Read the model definition and answer for the solid it produces. Units are mm, in the model's axes. A direction names the side the tool comes from. Round coordinates to 2 decimals unless told otherwise and drop trailing zeros. Loops run counter-clockwise (first coordinate to the right, second up) from the corner with the lowest first, then second, coordinate; pieces in that order, holes last. Notation, with made-up numbers: (85.25, 19) - (116.25, 19) arc R13 ccw to (116.25, 38) - close; hole circle Ø5 at (80, 77). An arc over 180 degrees is marked (long way). Answer as CSV lines item,"result".
```python
from build123d import *

# Parameters (mm, degrees)
F1_DEPTH = 57
F3_DEPTH = 20
F4_W     = 2.7
F4_H     = 7
F4_W_2   = 27.2
F5_DEPTH = 4.1
F6_DEPTH = 1.9


with BuildPart() as f1:
    # F0 (on Front) → F1 (new body)
    with BuildSketch(Plane.XZ):
        with BuildLine():
            Line((20.8, 15.8), (-20.8, 15.8))
            ThreePointArc((-20.8, 15.8), (-27.871068, 12.871068), (-30.8, 5.8))
            Line((-30.8, 5.8), (-30.8, 0))
            Line((-30.8, 0), (30.8, 0))
            Line((30.8, 0), (30.8, 5.8))
            ThreePointArc((30.8, 5.8), (27.871068, 12.871068), (20.8, 15.8))
        make_face()
    extrude(amount=F1_DEPTH)

    # F2 (on Right) → F3 (join, symmetric)
    with BuildSketch(Plane.YZ):
        with BuildLine():
            Line((0, 15), (0, 0))
            Line((0, 0), (0.6, 0))
            ThreePointArc((0.6, 0), (2.014214, 0.585786), (2.6, 2))
            Line((2.6, 2), (2.6, 13))
            ThreePointArc((2.6, 13), (2.014214, 14.414214), (0.6, 15))
            Line((0.6, 15), (0, 15))
        make_face()
    extrude(amount=F3_DEPTH, both=True)

    # F4 (on face) → F5 (cut)
    with BuildSketch(Plane.XZ.offset(57)):
        with Locations((-15.35, 7.7)):
            Rectangle(F4_W, F4_H)
        with Locations((-0.4, 7.7)):
            Rectangle(F4_W_2, F4_H)
        with Locations((14.55, 7.7)):
            Rectangle(F4_W, F4_H)
    extrude(amount=-F5_DEPTH, mode=Mode.SUBTRACT)

    # F4 (on face) → F6 (join)
    with BuildSketch(Plane.XZ.offset(57)):
        with Locations((-0.4, 7.7)):
            Rectangle(F4_W_2, F4_H)
    extrude(amount=-F6_DEPTH)


solid = f1.part
```
1) A cutting plane is placed at B-B, the plane z = 9.75. Determine the outline of the cut face in (x, y).
Entries:
outline,"(-29.99, -57) - (-16.7, -57) - (-16.7, -52.9) - (15.9, -52.9) - (15.9, -57) - (29.99, -57) - (29.99, 0) - (20, 0) - (20, 2.6) - (-20, 2.6) - (-20, 0) - (-29.99, 0) - close; (-14, -57) - (13.2, -57) - (13.2, -55.1) - (-14, -55.1) - close"
2) Each of these flat-tipped pins is pushed along its axis until it touches: P1, Ø6, axis at y = -10, z = 10, coming from the +X side; P2, Ø2, axis at y = -3.5, z = 10.5, coming from the -X side; P3, Ø2, axis at y = -56.5, z = 9.5, coming from the +X side. Where does it stop, or does it pass through?
Entries:
P1,"stops at x = 30.73"
P2,"stops at x = -30.09"
P3,"stops at x = 30.43"
3) A cutting plane is placed at D-D, the plane z = 3.5. Determine the outline of the cut face in (x, y), plus the area to 3 significant figures.
Entries:
outline,"(-30.8, -57) - (30.8, -57) - (30.8, 0) - (20, 0) - (20, 2.6) - (-20, 2.6) - (-20, 0) - (-30.8, 0) - close"
area,"3,620 mm^2"
4) A cutting plane is placed at C-C, the plane y = -33.5. Determine the outline of the cut face in (x, z), plus the area to 3 significant figures.
Entries:
outline,"(-30.8, 0) - (30.8, 0) - (30.8, 5.8) arc R10 ccw to (20.8, 15.8) - (-20.8, 15.8) arc R10 ccw to (-30.8, 5.8) - close"
area,"930 mm^2"
5) A tool of negligible diameter and unlimited length cuts with its end or side. For faces 5 (the face through (20, 1, 8)), 6 (the face through (-0.2, -54.5, 11.2)), 7 (the face through (15.9, -55, 8)), from which of +Z, -Z, +X, -X, +Y, -Y can it reach the whole face along a straight path? Write none if from no direction.
Entries:
face 5,"+Z, -Z, +X, +Y"
face 6,"none"
face 7,"-Y"
6) A cutting plane is placed at A-A, the plane x = 1. Determine the outline of the cut face in (y, z), plus the area to 3 significant figures.
Entries:
outline,"(-57, 0) - (0.6, 0) arc R2 ccw to (2.6, 2) - (2.6, 13) arc R2 ccw to (0.6, 15) - (0, 15) - (0, 15.8) - (-57, 15.8) - close; hole (-55.1, 4.2) - (-52.9, 4.2) - (-52.9, 11.2) - (-55.1, 11.2) - close"
area,"922 mm^2"
7) The mould has two halves that part along X. Classify faces 1 (the face through (-1, -52.9, 8)), 2 (the face through (0, -28, 0)), 3 (the face through (-14, -56, 8)), 4 (the face through (30.8, -28, 3)): pulls with the +X half, pulls with the -X half, needs draft (parallel to the pull), parting line crosses it, or undercut.
Entries:
face 1,"undercut"
face 2,"needs draft"
face 3,"undercut"
face 4,"pulls with the +X half"
8) Find the intervals of material crossed by line 1 (Z direction, x = 21, y = -19); line 2 (Y direction, x = 10, z = 10.5); line 3 (Y direction, x = 22, z = 14.75), in increasing order.
Entries:
line 1,"z = 0 to 15.8"
line 2,"y = -57 to -55.1, -52.9 to 2.6"
line 3,"y = -57 to 0"
